CAD build for the part. Positions are in the model's coordinates, mm. A direction names the side the tool comes from. Give positions to 0.01 mm unless a question says otherwise; leave off trailing zeros. Loops run counter-clockwise (first coordinate to the right, second up) from the corner with the lowest first, then second, coordinate; pieces in that order, holes last. Notation, with made-up numbers: M 46,76.5 L 84,76.5 A28 cw 84,97.5 Z; hole C 72,-36 d10. An arc over 180 degrees is marked long. Answer as CSV lines item,"result".
from build123d import *

# Parameters (mm, degrees)
EXTRUDE_1_DEPTH     = 36
SKETCH_2_R          = 4.25
CUT_EXTRUDE_1_DEPTH = 5
SKETCH_3_R          = 4.25
CUT_EXTRUDE_2_DEPTH = 5
FILLET_1_R          = 4
FILLET_2_R          = 1


with BuildPart() as part:
    # Эскиз1 → Бобышка-Вытянуть1 (new body, symmetric)
    with BuildSketch(Plane.XY):
        Polygon((0, 0), (42.426406871, 42.426406871), (45.961940777, 38.890872965), (22.85244978, 15.781381968), (27.318244413, 5), (60, 5), (60, 0), align=None)
        Polygon((20.556349186, 13.485281374), (24.071067812, 5), (12.071067812, 5), align=None, mode=Mode.SUBTRACT)
    extrude(amount=EXTRUDE_1_DEPTH, both=True)

    # Эскиз2 → Вырез-Вытянуть1 (cut)
    with BuildSketch(Plane(origin=(0, 0, 0), x_dir=(0, 0, 1), z_dir=(-0.707106781, 0.707106781, 0))):
        with Locations(Location((-20, 45, 0), (0, 0, 270))):  # turned: the seam where the file's is
            Circle(SKETCH_2_R)
        with Locations(Location((20, 45, 0), (0, 0, 270))):  # turned: the seam where the file's is
            Circle(SKETCH_2_R)
    extrude(amount=-CUT_EXTRUDE_1_DEPTH, mode=Mode.SUBTRACT)

    # Эскиз3 → Вырез-Вытянуть2 (cut)
    with BuildSketch(Plane.XZ):
        with Locations(Location((45, 15, 0), (0, 0, 270))):  # turned: the seam where the file's is
            Circle(SKETCH_3_R)
        with Locations(Location((45, -15, 0), (0, 0, 270))):  # turned: the seam where the file's is
            Circle(SKETCH_3_R)
    extrude(amount=-CUT_EXTRUDE_2_DEPTH, mode=Mode.SUBTRACT)

    # Скругление1
    fillet_1_edges = [part.edges().sort_by_distance(p)[0] for p in [
        (45.961940777, 38.890872965, 0),
        (60, 5, 0),
    ]]
    fillet(fillet_1_edges, radius=FILLET_1_R)

    # Скругление2
    fillet_2_edges = [part.edges().sort_by_distance(p)[0] for p in [
        (20.556349186, 13.485281374, 0),
        (12.071067812, 5, 0),
        (24.071067812, 5, 0),
    ]]
    fillet(fillet_2_edges, radius=FILLET_2_R)


solid = part.part
1) Flat gauge pins, fed straight in: pin 1 (2 mm diameter, centred on x = 17.5, y = 5.5, fed in from -Z); pin 2 (12 mm diameter, centred on y = 28.5, z = -2.5, fed in from +X); pin 3 (9 mm diameter, centred on x = 17, z = 13.5, fed in from +Y); pin 4 (3 mm diameter, centred on y = 38, z = 10.5, fed in from -X). Where does each tip first touch, or does it go through?
Answer below:
pin 1,"stops at z = -36"
pin 2,"stops at x = 41.57"
pin 3,"stops at y = 21.5"
pin 4,"stops at x = 36.5"
2) Band-saw the part on B-B on y = 8.5. Give the cut face in (x, z), and give its area (3 significant figures).
Answer below:
outline,"M 8.5,-36 L 15.57,-36 L 15.57,36 L 8.5,36 Z; M 22.62,-36 L 25.87,-36 L 25.87,36 L 22.62,36 Z"
area,"743 mm^2"
3) Band-saw the part on D-D on x = 26. Give the cut face in (y, z), and give its area (3 significant figures).
Answer below:
outline,"M 0,-36 L 8.18,-36 L 8.18,36 L 0,36 Z; M 18.93,-36 L 26,-36 L 26,36 L 18.93,36 Z"
area,"1,100 mm^2"
4) Band-saw the part on A-A on z = -14. Give the cut face in (x, y), and give its area (3 significant figures).
Answer below:
outline,"M 0,0 L 40.87,0 L 40.87,5 L 27.32,5 L 22.85,15.78 L 43.13,36.06 A4 ccw 43.13,41.72 L 42.43,42.43 Z; M 49.13,0 L 60,0 L 60,1 A4 ccw 56,5 L 49.13,5 Z; hole M 13.78,6.71 A1 ccw 14.49,5 L 22.57,5 A1 ccw 23.5,6.38 L 21.13,12.1 A1 ccw 19.5,12.43 Z"
area,"525 mm^2"
5) Drill centre lines: line 1 (Z direction, x = 37, y = 31); line 2 (Y direction, x = 45, z = 23.5); line 3 (X direction, y = 1.15, z = 15). Where is each one in solid material? Low to high. Write a range as from..to.
Answer below:
line 1,"z = -36..-22.93, -17.07..17.07, 22.93..36"
line 2,"y = 0..5"
line 3,"x = 1.15..40.75, 49.25..60"
6) Mould opens along X. For faces 5 (the face through (21, 21, 1)), 6 (the face through (16.6, 9.53, 0.5)), 7 (the face through (23, 12, -36)), 8 (the face through (44.305, 38.935, -0.504)) say: +X half, -X half, draft (parallel to the pull), parting line (faces both ways), or undercut.
Answer below:
face 5,"-X half"
face 6,"undercut"
face 7,"draft"
face 8,"+X half"
7) Band-saw the part on C-C on z = -28. Give the cut face in (x, y), and give its area (3 significant figures).
Answer below:
outline,"M 0,0 L 60,0 L 60,1 A4 ccw 56,5 L 27.32,5 L 22.85,15.78 L 43.13,36.06 A4 ccw 43.13,41.72 L 42.43,42.43 Z; hole M 13.78,6.71 A1 ccw 14.49,5 L 22.57,5 A1 ccw 23.5,6.38 L 21.13,12.1 A1 ccw 19.5,12.43 Z"
area,"566 mm^2"
8) Which spindle directions (+Z, -Z, +X, -X, +Y, -Y) get a long thin tool onto all of the face, cutting with end or side? Do faces 1 (the face through (40.85, 2.46, -14.08)), 2 (the face through (25.054, 10.466, 0.504)), 3 (the face through (13.57, 5.6, 0.5)), 4 (the face through (23, 12, 36)). Say none if no direction does.
Answer below:
face 1,"-Y"
face 2,"+Z, -Z, +X"
face 3,"+Z, -Z"
face 4,"+Z, +X, -X, +Y, -Y"
